Geometry check sheet. Reference: the model listing, model coordinates, mm. Give positions to 0.01 mm unless a question says otherwise; leave off trailing zeros. Order: outer loops, then holes, each group sorted by start corner. A loop starts at its lowest first (then second) coordinate and runs counter-clockwise, first axis right, second up. Notation, with made-up numbers: (40, 81) - (52, 81) arc R12 cw to (52, 101) - close; hole circle Ø2 at (48.25, -12). An arc over 180 degrees is marked (long way). Put each result on its own line as item: value. Start each with the question number.
```python
from build123d import *

# Parameters (mm, degrees)
SWEEP_THIN1_PROFILE_R   = 15.113
SWEEP_THIN1_PROFILE_R_2 = 13.589
SWEEP_THIN3_START       = 24.364184397
SWEEP_THIN3_OUTLINE_R   = 7.874
SWEEP_THIN3_OUTLINE_R_2 = 6.35
SWEEP_THIN3_DEPTH       = 152.4
CUT_EXTRUDE1_START      = -279.4
SKETCH47_R              = 13.589
CUT_EXTRUDE1_DEPTH      = 279.4
SKETCH48_R              = 13.589
CUT_EXTRUDE2_DEPTH      = 279.4


# Read off the part's stored shape, not the designer's step: Sweep-Thin3
with BuildPart() as part:
    # Sweep-Thin1: sweep along a path in Sketch1
    with BuildLine(Plane.XY) as sweep_thin1_path:
        Line((-567.536879433, 176.764184397), (270.663120567, 176.764184397))
        ThreePointArc((270.663120567, 176.764184397), (346.863120567, 100.564184397), (270.663120567, 24.364184397))
        Line((270.663120567, 24.364184397), (-567.536879433, 24.364184397))
    # Sweep-Thin1 profile (on start of the path) → Sweep-Thin1 (sweep)
    with BuildSketch(Plane(origin=(-567.536879433, 176.764184397, 0), x_dir=(0, 0, 1), z_dir=(1, 0, 0))):
        Circle(SWEEP_THIN1_PROFILE_R)
        Circle(SWEEP_THIN1_PROFILE_R_2, mode=Mode.SUBTRACT)
    sweep(path=sweep_thin1_path.line)

    # Sweep-Thin3 outline → Sweep-Thin3 (add)
    with BuildSketch(Plane(origin=(0, 0, 0), x_dir=(1, 0, 0), z_dir=(0, 1, 0)).offset(SWEEP_THIN3_START)):
        with Locations((-415.136879433, 0)):
            Circle(SWEEP_THIN3_OUTLINE_R)
        with Locations((-415.136879433, 0)):
            Circle(SWEEP_THIN3_OUTLINE_R_2, mode=Mode.SUBTRACT)
    extrude(amount=SWEEP_THIN3_DEPTH)

    # Sketch47 → Cut-Extrude1 (cut)
    with BuildSketch(Plane.ZY.offset(567.536879433).offset(CUT_EXTRUDE1_START)):
        with Locations(Location((0, 176.764184397, 0), (0, 0, 90))):
            Circle(SKETCH47_R)
    extrude(amount=CUT_EXTRUDE1_DEPTH, mode=Mode.SUBTRACT)

    # Sketch48 → Cut-Extrude2 (cut)
    with BuildSketch(Plane.ZY.offset(567.536879433)):
        with Locations(Location((0, 24.364184397, 0), (0, 0, 270))):
            Circle(SKETCH48_R)
    extrude(amount=-CUT_EXTRUDE2_DEPTH, mode=Mode.SUBTRACT)


solid = part.part
```
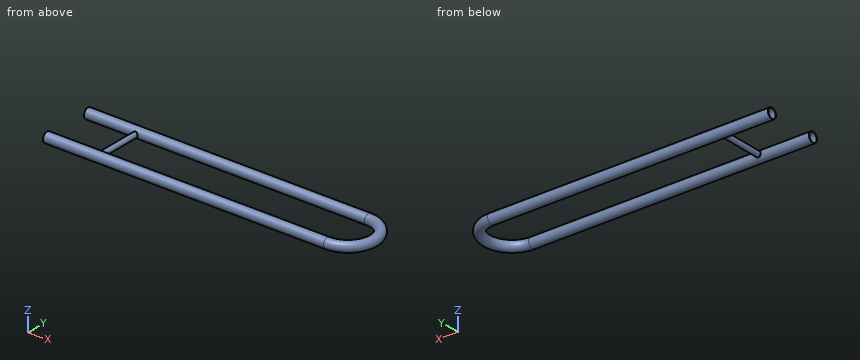
Item 1: Cross-section at C-C (y = 73). Count the separate pieces of the cut face and the enclosed holes in it, and give its area (3 significant figures).
Item 2: Gauge pin test, flat ends, axial feed: pin 1 Ø1.5 at (x, z) = (-30, 6.5) entering from +Y; pin 2 Ø6 at (y, z) = (125, 10) entering from -X; pin 3 Ø8 at (x, y) = (267, 35.5) entering from -Z. Record the tip position at first contact, or that the pin passes through.
Item 3: Thickness scan on line 1 along Y through (x, z) = (-78, 0); line 2 along Y through (x, z) = (0, -2); line 3 along Z through (x, y) = (-455.5, 175.5). Record the ranges inside material, lowest first.
Item 4: Cross-section at B-B (x = -358.5). Enter the section's corners in (y, z).
Recorded:
1. separate pieces: 2
1. enclosed holes: 2
1. area: 216 mm^2
2. pin 1: stops at y = 190.74
2. pin 2: stops at x = -418.74
2. pin 3: stops at z = -13.32
3. line 1: y = 9.25 to 10.78, 37.95 to 39.48, 161.65 to 163.18, 190.35 to 191.88
3. line 2: y = 9.38 to 10.92, 37.81 to 39.34, 161.78 to 163.32, 190.21 to 191.74
3. line 3: z = -15.06 to -13.53, 13.53 to 15.06
4. outline: circle Ø30.23 at (24.36, 0); circle Ø30.23 at (176.76, 0); hole circle Ø27.18 at (24.36, 0); hole circle Ø27.18 at (176.76, 0)
